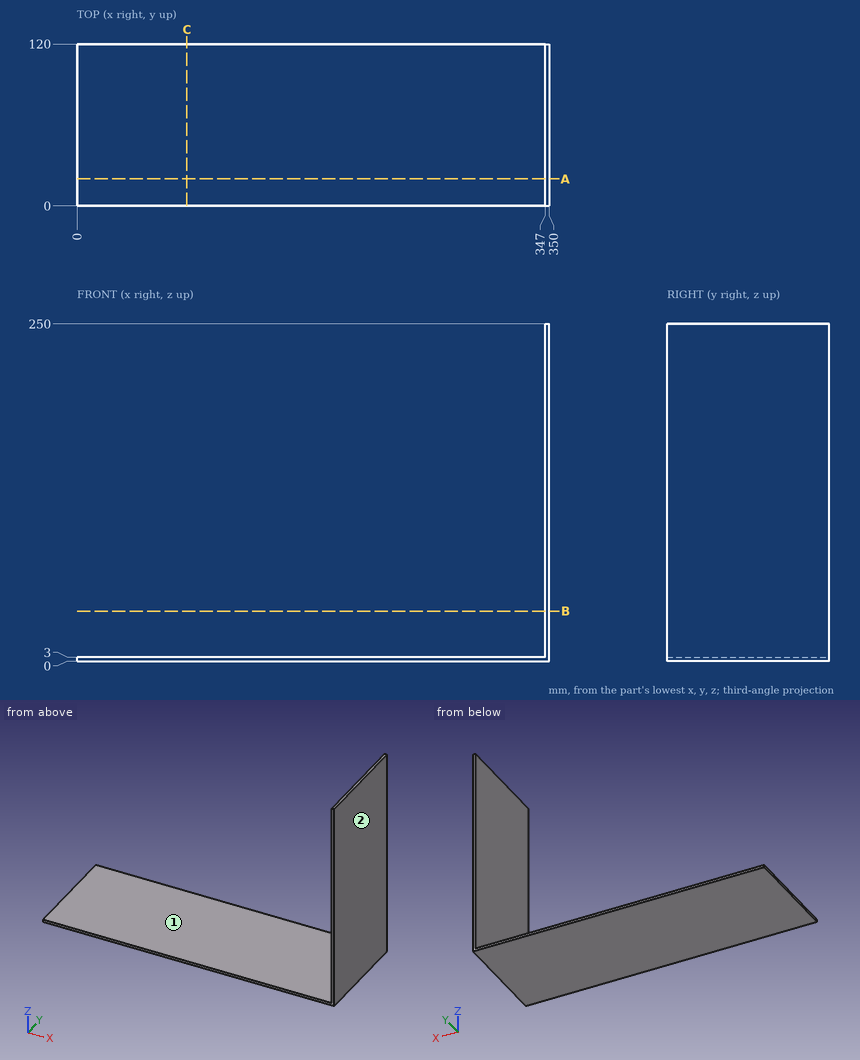
The figure shows three views and two pictorial views of one solid part (mm, origin at its lowest corner). Answer the questions. A direction names the side the tool comes from. Coordinates: 2 decimals unless noted, no trailing zeros. Loops run counter-clockwise (first coordinate to the right, second up) from the corner with the lowest first, then second, coordinate; pieces in that order, holes last. Notation, with made-up numbers: (55, -10.5) - (86, -10.5) arc R31 ccw to (86, 15.5) - close; hole circle Ø1 at (-37, 29.25). An arc over 180 degrees is marked (long way). Answer in a Markdown table with one row per item.
Q1. Find section A-A on y = 20. Write down the section's boundary in (x, z), plus the area to 3 significant figures.
Here are the results:
| item | result |
|---|---|
| outline | (0, 0) - (350, 0) - (350, 250) - (347, 250) - (347, 3) - (0, 3) - close |
| area | 1,790 mm^2 |
Q2. For the marked faces 1 and 2, determine the directions among +Z, -Z, +X, -X, +Y, -Y from which every point of the face is accessible in a straight line to the end or side of a thin tool.
Here are the results:
| item | result |
|---|---|
| face 1 | +Z, -X, +Y, -Y |
| face 2 | +Z, -Z, +X, +Y, -Y |
Q3. Find section C-C on x = 81.5. Write down the section's boundary in (y, z).
Here are the results:
| item | result |
|---|---|
| outline | (0, 0) - (120, 0) - (120, 3) - (0, 3) - close |
Q4. Find section B-B on z = 37. Write down the section's boundary in (x, y).
Here are the results:
| item | result |
|---|---|
| outline | (347, 0) - (350, 0) - (350, 120) - (347, 120) - close |
Q5. Given P1, Ø3, axis at y = 48, z = 170.5, coming from the -X side; P2, Ø10, axis at x = 279.5, y = 77.5, coming from the -Z side; P3, Ø1, axis at x = 78.5, y = 17, coming from the +Z side, each flat-ended and moving along its own axis, determine where each tip first touches the part or whether it passes through.
Here are the results:
| item | result |
|---|---|
| P1 | stops at x = 347 |
| P2 | stops at z = 0 |
| P3 | stops at z = 3 |
Q6. Straight lines are drawn through the part: line 1 along X through (y, z) = (80.5, 58); line 2 along Z through (x, y) = (168, 33.5). For each, find the intervals that lie inside material, in ascending order. Write a range as [from, to].
Here are the results:
| item | result |
|---|---|
| line 1 | x = [347, 350] |
| line 2 | z = [0, 3] |
